from build123d import *

# Parameters (mm, degrees)
F0_W     = 40.765519
F0_H     = 73.471674
F1_DEPTH = 5
F2_W     = 30.81081
F2_H     = 70
F3_DEPTH = 14
F4_W     = 35
F4_H     = 50.010137
F5_DEPTH = 8.5
F6_W     = 100
F6_H     = 24.910029
F7_DEPTH = 5
F8_R     = 1.85
F9_DEPTH = 25.4


with BuildPart() as f1:
    # F0 (on Top) → F1 (new body)
    with BuildSketch(Plane.XY):
        with Locations((4.975075, 16.320152)):
            Rectangle(F0_W, F0_H)
    extrude(amount=-F1_DEPTH)

    # F2 (on face) → F3 (join)
    with BuildSketch(Plane(origin=(0, 0, -5), x_dir=(1, 0, 0), z_dir=(0, 0, -1))):
        with Locations((5, -16.029622)):
            Rectangle(F2_W, F2_H)
        Polygon((10, -41.029622), (5, -41.029622), (0, -41.029622), (0, -22.373011), (10, -22.373011), align=None, mode=Mode.SUBTRACT)
        Polygon((0, 8.970378), (5, 8.970378), (10, 8.970378), (10, -11.889663), (0, -11.889663), align=None, mode=Mode.SUBTRACT)
    extrude(amount=F3_DEPTH)

    # F4 (on face) → F5 (cut)
    with BuildSketch(Plane(origin=(0, 0, -5), x_dir=(1, 0, 0), z_dir=(0, 0, -1))):
        with Locations((2.905405, -15.991903)):
            Rectangle(F4_W, F4_H)
    extrude(amount=F5_DEPTH, mode=Mode.SUBTRACT)

    # F6 (on face) → F7 (join)
    with BuildSketch(Plane(origin=(0, 0, -5), x_dir=(1, 0, 0), z_dir=(0, 0, -1))):
        with Locations((5.092296, -18.559826)):
            Rectangle(F6_W, F6_H)
    extrude(amount=-F7_DEPTH)

    # F8 (on face) → F9 (cut)
    with BuildSketch(Plane.XY):
        with Locations((-41.387634, 27.575926)):
            Circle(F8_R)
        with Locations((51.599746, 27.514396)):
            Circle(F8_R)
        with Locations((-41.413683, 9.564399)):
            Circle(F8_R)
        with Locations((51.624972, 9.70294)):
            Circle(F8_R)
    extrude(amount=-F9_DEPTH, mode=Mode.SUBTRACT)


solid = f1.part
Work out the finished part from the listing and answer in its coordinate system (mm). A direction names the side the tool comes from. Give positions to 0.01 mm unless a question says otherwise; leave off trailing zeros. Loops run counter-clockwise (first coordinate to the right, second up) from the corner with the lowest first, then second, coordinate; pieces in that order, holes last. Notation, with made-up numbers: (37, -11.5) -> (56, -11.5) arc R14 ccw to (56, 2.5) -> close; hole circle Ø10 at (20, 57). An arc over 180 degrees is marked (long way). Use a Markdown table: item, result. Add a question column.
1) For a pull along Y with two mould halves and no side action, classify faces 4 (the flat face through (5, 53.056, -2)), 5 (the flat face through (-10.405, 17, -15)), 6 (the flat face through (5, 16, -13.5)) as +Y half, -Y half, draft (parallel to the pull), parting line (faces both ways), or undercut.
2) The part is cut by section A-A, the plane x = 1.5. Determine the outline of the cut face in (y, z).
3) Consider line 1 along Z through (x, y) = (-6.5, 17); line 2 along Y through (x, z) = (-7.5, -10); line 3 along Z through (x, y) = (-32.5, 13.5). Determine where each line is inside the solid, lowest interval first.
4) Each of these flat-tipped pins is pushed along its axis until it touches: P1, Ø4, axis at x = 0.5, z = -10, coming from the -Y side; P2, Ø3, axis at x = -28, y = 5.5, coming from the -Z side; P3, Ø6, axis at x = -18, y = -8, coming from the +Z side; P4, Ø4.5, axis at y = -3, z = -17.5, coming from the -X side. Where does it stop, or does it pass through?
5) The part is cut by section D-D, the plane y = -1. Determine the outline of the cut face in (x, z), plus the area to 3 significant figures.
6) Which of the six approach directions +Z, -Z, +X, -X, +Y, -Y give full straight-line access (tool end or side, diameter ignored) to faces 1 (the flat face through (0, 32, -16)), 2 (the flat face through (-15.408, 42, -2)), 3 (the flat face through (5, -9.013, -9))?
7) The part is cut by section C-C, the plane z = -14.75. Determine the outline of the cut face in (x, y).
Reported:
| question | item | result |
|---|---|---|
| 1 | face 4 | +Y half |
| 1 | face 5 | draft |
| 1 | face 6 | undercut |
| 2 | outline | (-20.42, -5) -> (-18.97, -5) -> (-18.97, -19) -> (-8.97, -19) -> (-8.97, -13.5) -> (-9.01, -13.5) -> (-9.01, -5) -> (41.03, -5) -> (41.03, -19) -> (51.03, -19) -> (51.03, -5) -> (53.06, -5) -> (53.06, 0) -> (-20.42, 0) -> close; (11.89, -19) -> (22.37, -19) -> (22.37, -13.5) -> (11.89, -13.5) -> close |
| 3 | line 1 | z = -19 to -13.5, -5 to 0 |
| 3 | line 2 | y = -18.97 to -9.01, 41 to 51.03 |
| 3 | line 3 | z = -5 to 0 |
| 4 | P1 | stops at y = -18.97 |
| 4 | P2 | stops at z = -5 |
| 4 | P3 | stops at z = 0 |
| 4 | P4 | stops at x = -10.41 |
| 5 | outline | (-15.41, -5) -> (25.36, -5) -> (25.36, 0) -> (-15.41, 0) -> close; (-10.41, -19) -> (0, -19) -> (0, -13.5) -> (-10.41, -13.5) -> close; (10, -19) -> (20.41, -19) -> (20.41, -13.5) -> (10, -13.5) -> close |
| 5 | area | 318 mm^2 |
| 6 | face 1 | -Z |
| 6 | face 2 | +Z, -Z, -X, +Y |
| 6 | face 3 | +X, -X |
| 7 | outline | (-10.41, -18.97) -> (20.41, -18.97) -> (20.41, 51.03) -> (-10.41, 51.03) -> close; hole (0, -8.97) -> (10, -8.97) -> (10, 11.89) -> (0, 11.89) -> close; hole (0, 22.37) -> (10, 22.37) -> (10, 41.03) -> (0, 41.03) -> close |
